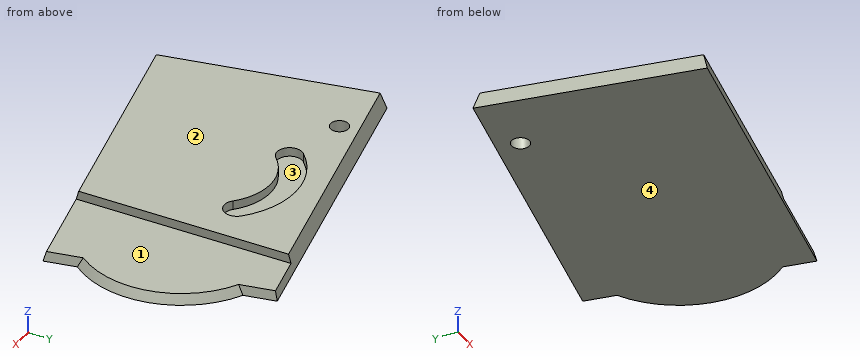
Autodesk Inventor part; units mm, degrees
ref_plane "YZ Plane" through (0, 0, 0) normal (1, 0, 0) x (0, 1, 0)
ref_plane "XZ Plane" through (0, 0, 0) normal (0, 1, 0) x (-1, 0, 0)
ref_plane "XY Plane" through (0, 0, 0) normal (0, 0, 1) x (1, 0, 0)
sketch "Sketch1" plane through (0, 0, 0) normal (0, 0, 1) x (1, 0, 0)
  line L0 (-76.521, -76.4496) -> (100, -41.2311)
  line L1 (100, -41.2311) -> (76.521, 76.4496)
  line L2 (76.521, 76.4496) -> (-100, 41.2311)
  line L3 (-100, 41.2311) -> (-76.521, -76.4496)
  line L4 (-76.521, -76.4496) -> (76.521, 76.4496) construction
  line L5 (100, -41.2311) -> (-100, 41.2311) construction
  point P0 (0, 0)
  point P1 (0, 0)
  dimension "d0" = 180
  dimension "d1" = 120
  dimension "d23" = 100
extrude "Extrusion1" add sketch "Sketch1" along normal blind 10 draft -15
sketch "Sketch2" plane through (0, 0, 0) normal (0, 0, 1) x (1, 0, 0)
  circle A0 centre (53.937, 10.7612) radius 55
  line L0 (100, -41.2311) -> (76.521, 76.4496) construction
  line L1 (0, 0) -> (88.2605, 17.6093) construction
  dimension "d1" = 120
  dimension "d4" = 110
  dimension "d5" = 55
extrude "Extrusion2" add sketch "Sketch2" along normal blind 10 draft -30
sketch "Sketch3" plane through (0, 0, 10) normal (0, 0, 1) x (1, 0, 0)
  line L0 (-74.4175, -73.2976) -> (-96.848, 39.1276)
  line L1 (-96.848, 39.1276) -> (74.4175, 73.2976)
  point P0 (0, 0)
  point P1 (-61.4584, 35.8123)
hole "Hole1" at (-61.4584, 35.8123, 10) direction (0, 0, -1) diameter 10 depth 18
sketch "Sketch4" plane through (0, 0, 10) normal (0, 0, 1) x (1, 0, 0)
  arc A0 (26.8701, 26.8701) -> (-26.8701, 26.8701) centre (0, 0) ccw construction
  arc A1 (31.8198, 31.8198) -> (-31.8198, 31.8198) centre (0, 0) ccw
  arc A2 (21.9203, 21.9203) -> (-21.9203, 21.9203) centre (0, 0) ccw
  arc A3 (21.9203, 21.9203) -> (31.8198, 31.8198) centre (26.8701, 26.8701) ccw
  arc A4 (-31.8198, 31.8198) -> (-21.9203, 21.9203) centre (-26.8701, 26.8701) ccw
  dimension "d18" = 90
  dimension "d19" = 7
  dimension "d20" = 38
extrude "Extrusion3" cut sketch "Sketch4" against normal blind 5
sketch "Sketch6" plane through (0, 0, 10) normal (0, 0, 1) x (1, 0, 0)
  line L0 (50.4655, 83.5966) -> (130.9866, 83.5966)
  line L1 (130.9866, 83.5966) -> (130.9866, -61.5092)
  line L2 (130.9866, -61.5092) -> (50.4655, -61.5092)
  line L3 (50.4655, -61.5092) -> (50.4655, 83.5966)
  point P0 (0, 0)
  dimension "d1" = 120
extrude "Extrusion4" cut sketch "Sketch6" against normal up to surface (5 mm away)
properties part number "Deo1 with Sketch"
Design review of the part built by this model. Coordinates are the model's own, in mm. Face numbers are marked on the shaded views. A direction names the side the tool comes from. Coordinates: 2 decimals unless noted, no trailing zeros. Loops run counter-clockwise (first coordinate to the right, second up) from the corner with the lowest first, then second, coordinate; pieces in that order, holes last.
Q1. We need section B-B on z = 7.5. State the section outline as (x, y) points, and give its area (3 significant figures).
Reported:
outline: (-97.64, 39.65) - (-74.94, -74.09) - (50.47, -49.06) - (50.47, 69.2) - close; hole circle Ø10 at (-61.46, 35.81); hole (-31.82, 31.82) arc R7 ccw to (-21.92, 21.92) arc R31 cw to (21.92, 21.92) arc R7 ccw to (31.82, 31.82) arc R45 ccw to start
area: 15,100 mm2
Q2. To check wall thickness, follow line 1 (X direction, y = 34.5, z = 5.5); line 2 (Z direction, x = 60, y = 49); line 3 (X direction, y = 34, z = 7). State the ranges of each line that lie inside material, in increasing order.
Reported:
line 1: x = -97.15 to -66.28, -56.63 to -28.89, 28.89 to 50.47
line 2: z = 0 to 5
line 3: x = -96.64 to -66.12, -56.8 to -29.48, 29.48 to 50.47
Q3. For pin 1 (3 mm diameter, centred on y = 15, z = 5, fed in from +X); pin 2 (2.5 mm diameter, centred on y = 31.5, z = 6.5, fed in from +X), all flat-tipped, find the tip position at first contact; note any pin that passes through.
Reported:
pin 1: stops at x = 106.75
pin 2: stops at x = 50.47
Q4. We need section A-A on x = -64. State the section outline as (y, z) points, and give its area (3 significant figures).
Reported:
outline: (-73.95, 0) - (31.51, 0) - (31.51, 10) - (-71.22, 10) - close; (40.12, 0) - (48.41, 0) - (45.68, 10) - (40.12, 10) - close
area: 1,110 mm2
Q5. We need section C-C on x = -26.87. State the section outline as (y, z) points.
Reported:
outline: (-66.54, 0) - (55.82, 0) - (53.09, 10) - (36.1, 10) - (36.1, 5) - (19.87, 5) - (19.87, 10) - (-63.81, 10) - close
Q6. The part is to be moulded in two halves that separate along X. For the marked faces 3 and 4, say which applies: +X half, -X half, draft (parallel to the pull), parting line (faces both ways), or undercut.
Reported:
face 3: undercut
face 4: draft
Q7. Tool access review of the marked faces 1 and 2: name each direction out of +Z, -Z, +X, -X, +Y, -Y from which nothing blocks a thin tool from reaching the whole face with its end or side.
Reported:
face 1: +Z, +X, +Y, -Y
face 2: +Z, +X, -X, +Y, -Y
Q8. We need section D-D on y = -56. State the section outline as (x, z) points.
Reported:
outline: (-80.6, 0) - (25.98, 0) - (12.28, 10) - (-77.87, 10) - close
